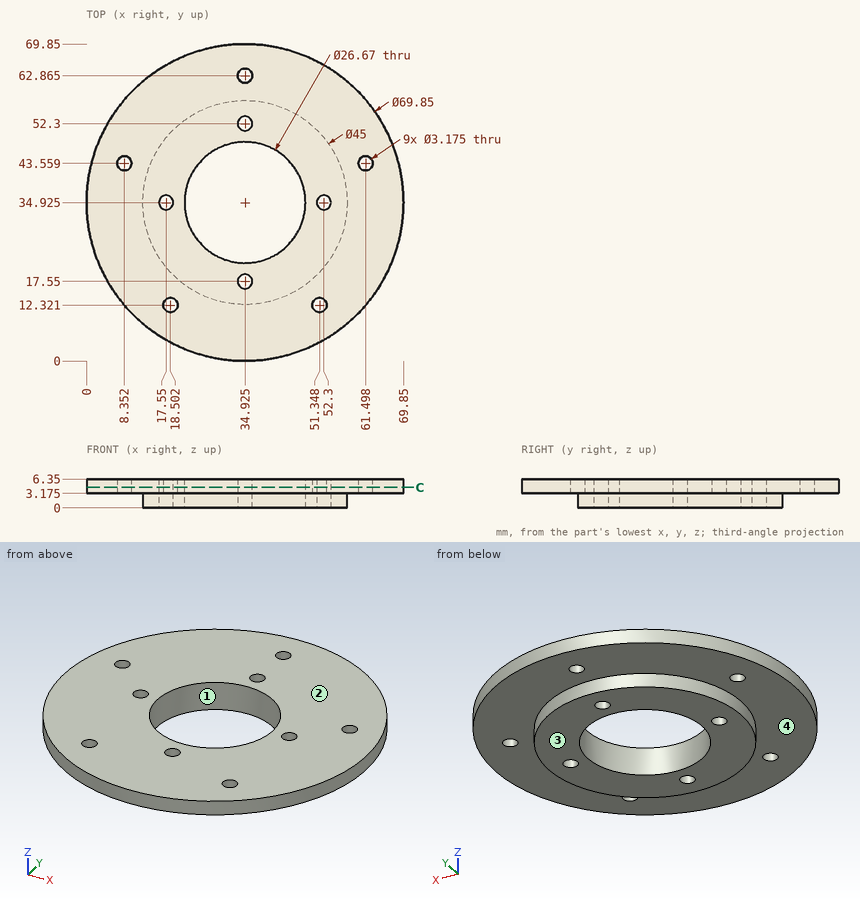
Print and shaded views of the part. All mm, measured from the part's lowest x, y and z. A direction names the side the tool comes from. Round coordinates to 2 decimals unless told otherwise and drop trailing zeros. Return JSON: item names as keys, results as strings. Group by question number.
Q1. Probe L1, parallel to Y at x = 40, z = 0.5 (1 decimal); L2, parallel to Y at x = 24, z = 3 (1 decimal); L3, parallel to X at y = 41, z = 5 (1 decimal). List the from-to ranges inside material, lowest first. Write a range as [from, to].
Q2. Saw through at C-C on z = 4.5. State how many separate pieces and enclosed holes the cut face has, plus the area to 3 significant figures.
Q3. Mould opens along X. For the marked faces 1 and 2 say: pulls with the +X half, pulls with the -X half, needs draft (parallel to the pull), parting line crosses it, or undercut.
Q4. Which spindle directions (+Z, -Z, +X, -X, +Y, -Y) get a long thin tool onto all of the face, cutting with end or side? Do the marked faces 3 and 4. Say none if no direction does.
Q5. Pin check, flat tips, straight feed: pin 1 (1.5 mm diameter, centred on y = 28.5, z = 3.5, fed in from +X); pin 2 (3.5 mm diameter, centred on x = 61.5, y = 43.56, fed in from +Z); pin 3 (5 mm diameter, centred on x = 51.35, y = 12.32, fed in from -Z) (1 decimal); pin 4 (1.5 mm diameter, centred on x = 49, z = 5, fed in from -Y). Stop position of each tip, or through.
Answer:
{
 "1": {"L1": "[13, 22.6], [47.3, 56.8]", "L2": "[15.3, 27.3], [42.6, 54.6]", "L3": "[0.5, 23.1], [46.8, 69.3]"},
 "2": {"separate pieces": "1", "enclosed holes": "10", "area": "3,200 mm2"},
 "3": {"face 1": "undercut", "face 2": "needs draft"},
 "4": {"face 3": "-Z, +X, -X, +Y, -Y", "face 4": "-Z"},
 "5": {"pin 1": "x = 69.39", "pin 2": "z = 6.35", "pin 3": "z = 3.2", "pin 4": "y = 2.64"}
}
